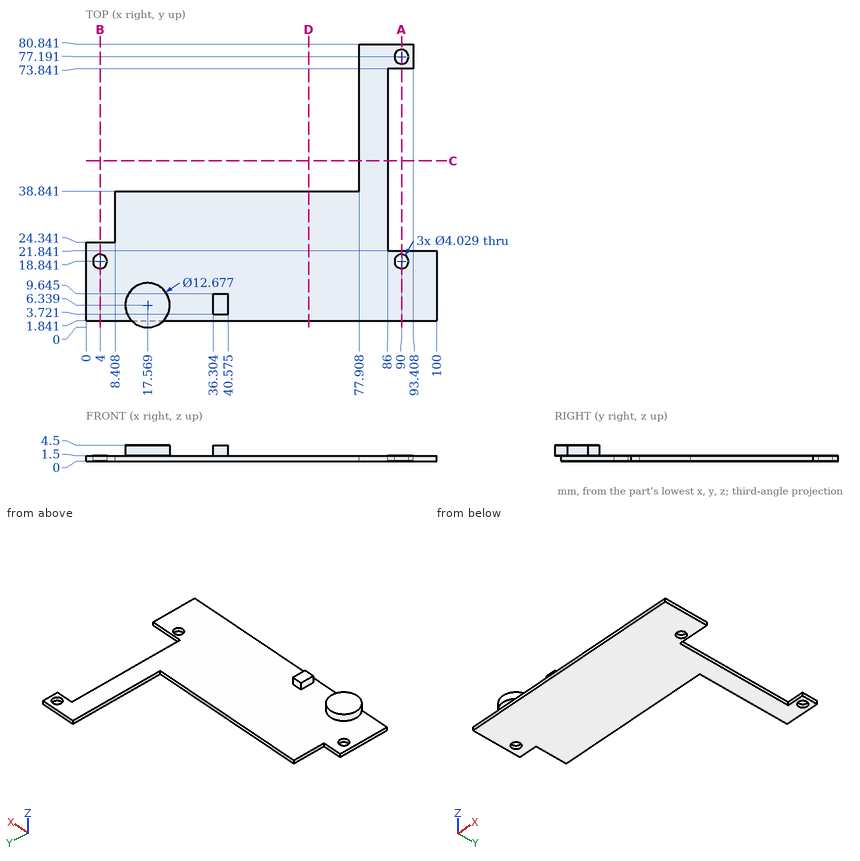
Can you work these out from the drawing? Everything is in mm from the part's minimum corner. Give positions to 0.01 mm unless a question says otherwise; leave off trailing zeros. Order: outer loops, then holes, each group sorted by start corner. A loop starts at its lowest first (then second) coordinate and runs counter-clockwise, first axis right, second up. Notation, with made-up numbers: M -27,-26 L 32,-26 A24 cw 32,-6 Z; hole C -19,80 d4. An arc over 180 degrees is marked long. Use a Markdown table: item, result. Add a question column.
1. Suppose I cut it at A-A (x = 90). List the corners of the cut face in (y, z) for me (1 decimal).
2. I need wall thicknesses on probe 1 along Y at (x, z) = (90, 1.1) (1 decimal); probe 2 along Y at (x, z) = (4, 1.05) (1 decimal); probe 3 along Y at (x, z) = (37, 3.95) (1 decimal). Which ranges of each line are inside material? Lowest first, please. Write a range as from..to.
3. For pin 1 Ø0.8 at (y, z) = (78.5, 0.5) entering from +X; pin 2 Ø1.6 at (x, z) = (53.5, 0.5) entering from +Y; pin 3 Ø3.5 at (x, y) = (90, 77.19) entering from +Z; pin 4 Ø1.2 at (y, z) = (34.5, 1) entering from -X, each with a flat end and sliding along its axis, tell me the tip position at first contact or that it passes through.
4. Suppose I cut it at B-B (x = 4). List the corners of the cut face in (y, z) for me (1 decimal), and give its area (3 significant figures).
5. Suppose I cut it at D-D (x = 63.5). List the corners of the cut face in (y, z) for me.
6. Suppose I cut it at C-C (y = 47.5). List the corners of the cut face in (x, z) for me.
Results list:
| question | item | result |
|---|---|---|
| 1 | outline | M 1.8,0 L 16.8,0 L 16.8,1.5 L 1.8,1.5 Z; M 20.9,0 L 21.8,0 L 21.8,1.5 L 20.9,1.5 Z; M 73.8,0 L 75.2,0 L 75.2,1.5 L 73.8,1.5 Z; M 79.2,0 L 80.8,0 L 80.8,1.5 L 79.2,1.5 Z |
| 2 | probe 1 | y = 1.8..16.8, 20.9..21.8, 73.8..75.2, 79.2..80.8 |
| 2 | probe 2 | y = 1.8..16.8, 20.9..24.3 |
| 2 | probe 3 | y = 3.7..9.6 |
| 3 | pin 1 | stops at x = 93.41 |
| 3 | pin 2 | stops at y = 38.84 |
| 3 | pin 3 | passes through |
| 3 | pin 4 | stops at x = 8.41 |
| 4 | outline | M 1.8,0 L 16.8,0 L 16.8,1.5 L 1.8,1.5 Z; M 20.9,0 L 24.3,0 L 24.3,1.5 L 20.9,1.5 Z |
| 4 | area | 27.7 mm² |
| 5 | outline | M 1.84,0 L 38.84,0 L 38.84,1.5 L 1.84,1.5 Z |
| 6 | outline | M 77.91,0 L 86,0 L 86,1.5 L 77.91,1.5 Z |
